Design review of the part built by this model. Coordinates are the model's own, in mm. A direction names the side the tool comes from. Coordinates: 2 decimals unless noted, no trailing zeros. Order: outer loops, then holes, each group sorted by start corner. A loop starts at its lowest first (then second) coordinate and runs counter-clockwise, first axis right, second up. Notation, with made-up numbers: M 80.25,-32.75 L 99.25,-32.75 A20 cw 99.25,-6.75 Z; hole C 19,36 d6. An arc over 180 degrees is marked long. Answer in a Markdown table with one row per item.
from build123d import *

# Parameters (mm, degrees)
SKETCH_2_R      = 1
SKETCH_2_R_2    = 1.5
SKETCH_2_R_3    = 3
EXTRUDE_1_DEPTH = 2


with BuildPart() as part:
    # 草图2 → 凸台-拉伸1 (new body)
    with BuildSketch(Plane.XY):
        with BuildLine():
            Line((0, 4), (34, 4))
            ThreePointArc((34, 4), (38, 0), (34, -4))
            Line((34, -4), (0, -4))
            Line((0, -4), (-6, -4))
            Line((-6, -4), (-6, 4))
            Line((-6, 4), (0, 4))
        make_face()
        with Locations((-4, 2)):
            Circle(SKETCH_2_R, mode=Mode.SUBTRACT)
        Circle(SKETCH_2_R_2, mode=Mode.SUBTRACT)
        with Locations((34, 0)):
            Circle(SKETCH_2_R_3, mode=Mode.SUBTRACT)
        with Locations((-4, -2)):
            Circle(SKETCH_2_R, mode=Mode.SUBTRACT)
        with BuildLine():
            Line((10, 2), (24, 2))
            ThreePointArc((24, 2), (26, 0), (24, -2))
            Line((24, -2), (10, -2))
            ThreePointArc((10, -2), (8, 0), (10, 2))
        make_face(mode=Mode.SUBTRACT)
    extrude(amount=EXTRUDE_1_DEPTH)


solid = part.part
(1) Add section C-C, the plane z = 1. Give the boundary of the cut face in (x, y), and give its area (3 significant figures).
Return value:
| item | result |
|---|---|
| outline | M -6,-4 L 34,-4 A4 ccw 34,4 L -6,4 Z; hole C -4,-2 d2; hole C -4,2 d2; hole C 0,0 d3; hole M 10,-2 L 24,-2 A2 ccw 24,2 L 10,2 A2 ccw Z; hole C 34,0 d6 |
| area | 235 mm2 |
(2) Add section D-D, the plane y = 2.5. Give the boundary of the cut face in (x, z).
Return value:
| item | result |
|---|---|
| outline | M -6,0 L -4.87,0 L -4.87,2 L -6,2 Z; M -3.13,0 L 32.34,0 L 32.34,2 L -3.13,2 Z; M 35.66,0 L 37.12,0 L 37.12,2 L 35.66,2 Z |
(3) For line 1 along Y through (x, z) = (-4, 0.7); line 2 along X through (y, z) = (-2.5, 0.3); line 3 along Y through (x, z) = (12, 1.7), list the stretches that pass through material, from the lowest coordinate up. Write a range as from..to.
Return value:
| item | result |
|---|---|
| line 1 | y = -4..-3, -1..1, 3..4 |
| line 2 | x = -6..-4.87, -3.13..32.34, 35.66..37.12 |
| line 3 | y = -4..-2, 2..4 |
(4) Draft analysis for pull direction X (two halves, no side actions). For faces 3 (the flat face through (17, 2, 1)), 4 (the flat face through (-6, 0, 1)), 5 (the flat face through (14, -4, 1)), state which applies: pulls with the +X half, pulls with the -X half, needs draft (parallel to the pull), parting line crosses it, or undercut.
Return value:
| item | result |
|---|---|
| face 3 | undercut |
| face 4 | pulls with the -X half |
| face 5 | needs draft |
(5) Add section A-A, the plane y = 0. Give the boundary of the cut face in (x, z).
Return value:
| item | result |
|---|---|
| outline | M -6,0 L -1.5,0 L -1.5,2 L -6,2 Z; M 1.5,0 L 8,0 L 8,2 L 1.5,2 Z; M 26,0 L 31,0 L 31,2 L 26,2 Z; M 37,0 L 38,0 L 38,2 L 37,2 Z |
(6) For faces 1 (the cylindrical face through (26, 0, 1)), 2 (the flat face through (16, -3, 2)), list the 3-axis set-ups (+Z, -Z, +X, -X, +Y, -Y) from which the entire face can be reached by the end or side of a thin tool; tool diameter is ignored.
Return value:
| item | result |
|---|---|
| face 1 | +Z, -Z |
| face 2 | +Z, +X, -X, +Y, -Y |
(7) Add section B-B, the plane x = 0. Give the boundary of the cut face in (y, z).
Return value:
| item | result |
|---|---|
| outline | M -4,0 L -1.5,0 L -1.5,2 L -4,2 Z; M 1.5,0 L 4,0 L 4,2 L 1.5,2 Z |
